The model under review builds one solid part; all positions refer to its coordinate system, in mm. A direction names the side the tool comes from. Give positions to 0.01 mm unless a question says otherwise; leave off trailing zeros. Order: outer loops, then holes, each group sorted by start corner. A loop starts at its lowest first (then second) coordinate and runs counter-clockwise, first axis right, second up.
Autodesk Inventor part; units mm, degrees
ref_plane "Work Plane1" through (-54.875, -108.1, -1.5875) normal (1, 0, 0) x (0, 1, 0)
ref_plane "YZ Plane" through (0, 0, 0) normal (1, 0, 0) x (0, 1, 0)
ref_plane "XZ Plane" through (0, 0, 0) normal (0, 1, 0) x (-1, 0, 0)
sketch "Sketch1" plane through (0, 0, 0) normal (0, 0, 1) x (1, 0, 0)
  line L0 (-1.5875, 0) -> (-1.5875, -108.1)
  line L1 (-54.875, 0) -> (-1.5875, 0)
  line L2 (-54.875, 0) -> (-54.875, -59)
  line L3 (-54.875, -59) -> (-18.9375, -59)
  arc A0 (-18.9375, -75) -> (-18.9375, -59) centre (-18.9375, -67) ccw
  line L4 (-18.9375, -75) -> (-54.875, -75)
  line L5 (-54.875, -75) -> (-54.875, -108.1)
  line L6 (-54.875, -108.1) -> (-1.5875, -108.1)
  circle A1 centre (-18.9375, -67) radius 2
  circle A2 centre (-18.9375, -67) radius 2
  circle A3 centre (-18.9375, -67) radius 7.5
  line L7 (-6.1875, -79.75) -> (-31.6875, -79.75) construction
  line L8 (-31.6875, -79.75) -> (-31.6875, -54.25) construction
  line L9 (-31.6875, -54.25) -> (-6.1875, -54.25) construction
  line L10 (-6.1875, -54.25) -> (-6.1875, -79.75) construction
  line L11 (-18.9375, -79.75) -> (-18.9375, -54.25) construction
  line L12 (-31.6875, -67) -> (-6.1875, -67) construction
  circle A4 centre (-6.1875, -79.75) radius 1.5
  circle A5 centre (-31.6875, -79.75) radius 1.5
  circle A6 centre (-31.6875, -54.25) radius 1.5
  circle A7 centre (-6.1875, -54.25) radius 1.5
  circle A8 centre (-6.1875, -79.75) radius 2.6 construction
  circle A9 centre (-31.6875, -79.75) radius 2.6 construction
  circle A10 centre (-31.6875, -54.25) radius 2.6 construction
  circle A11 centre (-6.1875, -54.25) radius 2.6 construction
  line L13 (-3.5875, -79.75) -> (-3.5875, -54.25) construction
  arc A12 (-8.0517, -82.7122) -> (-3.5875, -77.4069) centre (-6.1875, -79.75) ccw
  arc A13 (-34.6497, -77.8858) -> (-29.8233, -82.7122) centre (-31.6875, -79.75) ccw
  arc A14 (-29.8233, -51.2878) -> (-34.6497, -56.1142) centre (-31.6875, -54.25) ccw
  arc A15 (-3.5875, -56.5931) -> (-8.0517, -51.2878) centre (-6.1875, -54.25) ccw
  line L14 (-8.0517, -82.7122) -> (-17.8722, -76.532)
  line L15 (-34.6497, -56.1142) -> (-28.4695, -65.9347)
  line L16 (-34.6497, -77.8858) -> (-28.4695, -68.0653)
  line L17 (-3.2253, -56.1142) -> (-9.4055, -65.9347)
  line L18 (-3.2253, -77.8858) -> (-9.4055, -68.0653)
  line L19 (-29.8233, -51.2878) -> (-20.0028, -57.468)
  line L20 (-8.0517, -51.2878) -> (-17.8722, -57.468)
  line L21 (-20.3773, -59) -> (-20.6867, -59.1936)
  line L22 (-29.8233, -82.7122) -> (-20.0028, -76.532)
  arc A16 (-20.0028, -57.468) -> (-17.8722, -57.468) centre (-18.9375, -55.7753) ccw
  arc A17 (-28.4695, -68.0653) -> (-28.4695, -65.9347) centre (-30.1622, -67) ccw
  arc A18 (-17.8722, -76.532) -> (-20.0028, -76.532) centre (-18.9375, -78.2247) ccw
  arc A19 (-9.4055, -65.9347) -> (-9.4055, -68.0653) centre (-7.7128, -67) ccw
  circle A20 centre (-18.9375, -67) radius 2.5
  circle A21 centre (-31.6875, -54.25) radius 2.6
  circle A22 centre (-6.1875, -79.75) radius 2.6
  circle A23 centre (-6.1875, -54.25) radius 2.6
  circle A24 centre (-31.6875, -79.75) radius 2.6
  point P0 (0, 0)
  point P1 (-27.7991, -67)
  point P2 (-10.0759, -67)
  point P3 (-18.9375, -58.1384)
  point P4 (-18.9375, -75.8616)
  dimension "d2" = 5.2
  dimension "d1" = 3
  dimension "d4" = 2
  dimension "d5" = 2
  dimension "d6" = 2
  dimension "d9" = 0.5
extrude "Extrusion1" add sketch "Sketch1" along normal blind 4 contours L15 A14 L19 A16 L20 A15 L17 A19 L18 A12 L14 A18 L22 A13 L16 L4 A0 L3 | L3 A0 L4 L16 A17 L15 | A3 | A21 | A22 | A23 | A24
sketch "Sketch2" plane through (0, 0, 0) normal (0, 0, -1) x (-1, 0, 0)
  circle A0 centre (18.9375, -67) radius 7.5
  point P0 (0, 0)
extrude "Extrusion2" add sketch "Sketch2" along normal blind 1
sketch "Sketch3" plane through (0, 0, 0) normal (0, 0, -1) x (-1, 0, 0)
  line L0 (1.5875, 0) -> (1.5875, -108.1)
  line L1 (54.875, 0) -> (1.5875, 0)
  line L2 (54.875, 0) -> (54.875, -59)
  line L3 (54.875, -59) -> (18.9375, -59)
  arc A0 (18.9375, -59) -> (18.9375, -75) centre (18.9375, -67) ccw
  line L4 (18.9375, -75) -> (54.875, -75)
  line L5 (54.875, -75) -> (54.875, -108.1)
  line L6 (54.875, -108.1) -> (1.5875, -108.1)
  circle A1 centre (18.9375, -67) radius 7.5
  arc A2 (18.9375, -59) -> (18.9375, -75) centre (18.9375, -67) ccw
  circle A3 centre (18.9375, -67) radius 2.5
  arc A4 (22.7022, -74.0588) -> (22.7022, -59.9412) centre (18.9375, -67) ccw
  line L7 (53.2875, -108.1) -> (53.2875, 0)
  line L8 (54.875, 0) -> (54.875, -108.1)
  line L9 (53.2875, -59) -> (22.9375, -59)
  line L10 (18.9375, -59) -> (18.9375, -75)
  line L11 (22.9375, -75) -> (53.2875, -75)
  line L12 (53.2875, -75) -> (53.2875, -59)
  arc A5 (22.9375, -59) -> (22.7022, -59.9412) centre (22.9375, -59.5) ccw
  arc A6 (22.7022, -74.0588) -> (22.9375, -75) centre (22.9375, -74.5) ccw
  circle A7 centre (31.6875, -54.25) radius 2.6
  circle A8 centre (6.1875, -79.75) radius 2.6
  circle A9 centre (6.1875, -54.25) radius 2.6
  circle A10 centre (31.6875, -79.75) radius 2.6
  point P0 (0, 0)
  dimension "d12" = 0.5
extrude "Extrusion3" add sketch "Sketch3" along normal blind 2 contours L7 L4 A6 A4 A5 L3
sketch "Sketch4" plane through (-53.2875, -75, 0) normal (-1, 0, 0) x (0, 0, 1)
  line L0 (-1.5875, 75) -> (-1.5875, -33.1)
  line L1 (0, -33.1) -> (0, 75)
  line L2 (0, 15.0588) -> (0, 16)
  line L3 (0, 0) -> (-2, 0)
  line L4 (0, 16) -> (-1.5875, 16)
  line L5 (-1.5875, 16) -> (-1.5875, 0)
  line L6 (-1.5875, 0) -> (0, 0)
  line L7 (0, 0) -> (0, 16)
ref_plane "Work Plane1" through (-54.875, -108.1, -1.5875) normal (1, 0, 0) x (0, 1, 0)
extrude "Extrusion4" add sketch "Sketch4" along normal up to surface (1.5875 mm away)
sketch "Sketch5" plane through (0, 0, 4) normal (0, 0, 1) x (1, 0, 0)
  arc A0 (-28.4695, -68.0653) -> (-28.4695, -65.9347) centre (-30.1622, -67) ccw
  line L0 (-28.4695, -68.0653) -> (-34.6497, -77.8858)
  arc A1 (-34.6497, -77.8858) -> (-29.8233, -82.7122) centre (-31.6875, -79.75) ccw
  line L1 (-29.8233, -82.7122) -> (-20.0028, -76.532)
  arc A2 (-17.8722, -76.532) -> (-20.0028, -76.532) centre (-18.9375, -78.2247) ccw
  line L2 (-17.8722, -76.532) -> (-8.0517, -82.7122)
  arc A3 (-8.0517, -82.7122) -> (-3.2253, -77.8858) centre (-6.1875, -79.75) ccw
  line L3 (-3.2253, -77.8858) -> (-9.4055, -68.0653)
  arc A4 (-9.4055, -65.9347) -> (-9.4055, -68.0653) centre (-7.7128, -67) ccw
  line L4 (-9.4055, -65.9347) -> (-3.2253, -56.1142)
  arc A5 (-3.2253, -56.1142) -> (-8.0517, -51.2878) centre (-6.1875, -54.25) ccw
  line L5 (-8.0517, -51.2878) -> (-17.8722, -57.468)
  arc A6 (-20.0028, -57.468) -> (-17.8722, -57.468) centre (-18.9375, -55.7753) ccw
  line L6 (-20.0028, -57.468) -> (-29.8233, -51.2878)
  arc A7 (-29.8233, -51.2878) -> (-34.6497, -56.1142) centre (-31.6875, -54.25) ccw
  line L7 (-34.6497, -56.1142) -> (-28.4695, -65.9347)
  circle A8 centre (-18.9375, -67) radius 2.5
  circle A9 centre (-6.1875, -54.25) radius 1.5
  circle A10 centre (-31.6875, -54.25) radius 1.5
  circle A11 centre (-31.6875, -79.75) radius 1.5
  circle A12 centre (-6.1875, -79.75) radius 1.5
  circle A13 centre (-31.6875, -79.75) radius 3.5
  circle A14 centre (-31.6875, -54.25) radius 1.5
  circle A15 centre (-31.6875, -54.25) radius 3.5
  circle A16 centre (-6.1875, -79.75) radius 3.5
  arc A17 (-3.2253, -56.1142) -> (-8.0517, -51.2878) centre (-6.1875, -54.25) ccw
  circle A18 centre (-6.1388, -54.2188) radius 3.5
  point P0 (0, 0)
  point P1 (-34.6497, -56.1142)
  point P2 (-29.8233, -51.2878)
  point P3 (-2.2565, -55.1629)
  point P4 (-3.2253, -77.8858)
  point P5 (-8.0517, -82.7122)
  point P6 (-29.8233, -82.7122)
  point P7 (-3.4179, -56.4203)
extrude "Extrusion5" cut sketch "Sketch5" against normal blind 2 contours A13 A1 | A7 A15 | A16 A3 | A5 L4 A18 picked at (-4.1737, -56.2279)
fillet "Fillet1" radius 1 10 edges at (-8.0517, -82.7122, 3) (-3.2253, -77.8858, 3) (-3.2253, -56.1142, 1) (-8.0517, -51.2878, 1) (-29.8233, -51.2878, 3) (-34.6497, -56.1142, 3) (-34.6497, -77.8858, 3) (-29.8233, -82.7122, 3) (-3.4179, -56.4203, 3) (-8.0517, -51.2878, 3)
sketch "Sketch6" plane through (0, 0, 0) normal (0, 0, 1) x (1, 0, 0)
  line L0 (-32.8336, -59) -> (-28.4695, -65.9347)
  line L1 (-32.8336, -59) -> (-54.875, -59)
  line L2 (-54.875, -75) -> (-54.875, -59)
  line L3 (-32.8336, -75) -> (-54.875, -75)
  line L4 (-28.4695, -68.0653) -> (-32.8336, -75)
  arc A0 (-28.4695, -68.0653) -> (-28.4695, -65.9347) centre (-30.1622, -67) ccw
  line L5 (-53.2875, 0) -> (-53.2875, -108.1)
  line L6 (-35.6304, -72.5101) -> (-44.525, -72.5101)
  line L7 (-46.525, -70.5101) -> (-46.525, -63.4899)
  line L8 (-44.525, -61.4899) -> (-35.6304, -61.4899)
  line L9 (-33.6304, -63.4899) -> (-33.6304, -70.5101)
  line L10 (-28.1622, -67) -> (-54.875, -67) construction
  line L11 (-54.875, -59) -> (-54.875, -75) construction
  line L12 (-48.525, -39.75) -> (-48.525, -93.75) construction
  arc A1 (-35.6304, -72.5101) -> (-33.6304, -70.5101) centre (-35.6304, -70.5101) ccw
  arc A2 (-46.525, -70.5101) -> (-44.525, -72.5101) centre (-44.525, -70.5101) ccw
  arc A3 (-44.525, -61.4899) -> (-46.525, -63.4899) centre (-44.525, -63.4899) ccw
  arc A4 (-33.6304, -63.4899) -> (-35.6304, -61.4899) centre (-35.6304, -63.4899) ccw
  point P0 (0, 0)
  dimension "d20" = 2
  dimension "d21" = 2
extrude "Extrusion6" cut sketch "Sketch6" against normal through all contours L6 A2 L7 A3 L8 A4 L9 A1
properties part number "TurretBase"
Item 1: Take a section at B-B (z = 2.8). Give the boundary of the cut face in (x, y).
Values found:
outline: (-32.66, -74.72) arc R1 ccw to (-31.78, -76.25) arc R3.5 cw to (-28.19, -79.85) arc R1 ccw to (-26.66, -80.72) - (-20, -76.53) arc R2 cw to (-17.87, -76.53) - (-11.22, -80.72) arc R1 ccw to (-9.69, -79.85) arc R3.5 cw to (-6.09, -76.25) arc R1 ccw to (-5.22, -74.72) - (-9.41, -68.07) arc R2 cw to (-9.41, -65.93) - (-5.2, -59.25) arc R1 ccw to (-6.07, -57.72) arc R3.5 cw to (-9.64, -54.12) arc R1 ccw to (-11.17, -53.25) - (-17.87, -57.47) arc R2 cw to (-20, -57.47) - (-26.66, -53.28) arc R1 ccw to (-28.19, -54.15) arc R3.5 cw to (-31.78, -57.75) arc R1 ccw to (-32.66, -59.28) - (-28.47, -65.93) arc R2 cw to (-28.47, -68.07) - close; hole circle Ø5 at (-18.94, -67)
Item 2: Draft analysis for pull direction X (two halves, no side actions). For faces 6 (the cylindrical face through (-34.2, -62.09, -0.99)), 7 (the flat face through (-6.96, -71.95, 1.97)), 8 (the cylindrical face through (-32.88, -53.34, 0.99)), 9 (the flat face through (-39, -75, -1)), state which applies: released by +X, released by -X, zero draft, split by the parting line, or undercut.
Values found:
face 6: undercut
face 7: released by +X
face 8: undercut
face 9: zero draft
Item 3: Clearance check with flat-ended pins moving along their axes: pin 1 Ø1.8 at (x, y) = (-31.69, -79.75) entering from +Z; pin 2 Ø2 at (y, z) = (-70.5, 2) entering from -X; pin 3 Ø0.6 at (x, z) = (-39, -0.5) entering from +Y; pin 4 Ø4.5 at (x, y) = (-21, -64.5) entering from -Z. State where each tip first meets the part, or that it passes through.
Values found:
pin 1: passes through
pin 2: stops at x = -30.63
pin 3: stops at y = -59
pin 4: stops at z = -1
Item 4: For faces 1 (the flat face through (-33.63, -67, -1)), 2 (the flat face through (-6.96, -62.05, 1.97)), 3 (the flat face through (-23.89, -55.02, 1.97)), 4 (the cylindrical face through (-28.162, -66.984, 1.972)), 5 (the flat face through (-19, -67, 0)), list the 3-axis set-ups (+Z, -Z, +X, -X, +Y, -Y) from which the entire face can be reached by the end or side of a thin tool; tool diameter is ignored.
Values found:
face 1: +Z, -Z
face 2: +Z, -Z, +X
face 3: +Z, -Z, +Y
face 4: +Z, -X
face 5: +Z
Item 5: Take a section at A-A (y = -67). Give the boundary of the cut face in (x, z) (1 decimal), and give its area (3 significant figures).
Values found:
outline: (-54.9, -1.6) - (-53.3, -1.6) - (-53.3, -2) - (-46.5, -2) - (-46.5, 0) - (-54.9, 0) - close; (-33.6, -2) - (-26.9, -2) - (-26.9, 0) - (-26.4, 0) - (-26.4, -1) - (-11.4, -1) - (-11.4, 0) - (-9.7, 0) - (-9.7, 4) - (-16.4, 4) - (-16.4, 0) - (-21.4, 0) - (-21.4, 4) - (-28.2, 4) - (-28.2, 0) - (-33.6, 0) - close
area: 98.2 mm2
Item 6: Take a section at C-C (x = -13). Give the boundary of the cut face in (y, z), and give its area (3 significant figures).
Values found:
outline: (-79.6, 0) - (-71.58, 0) - (-71.58, -1) - (-62.42, -1) - (-62.42, 0) - (-54.4, 0) - (-54.4, 4) - (-79.6, 4) - close
area: 110 mm2
Item 7: Take a section at D-D (x = -49.5). Give the boundary of the cut face in (y, z).
Values found:
outline: (-75, -2) - (-59, -2) - (-59, 0) - (-75, 0) - close
Item 8: For line 1 (Y direction, x = -19, z = 0.7); line 2 (Z direction, x = -12, y = -54.5); line 3 (Z direction, x = -52, y = -73.5), list the stretches that pass through material, from the lowest coordinate up.
Values found:
line 1: y = -76.23 to -69.5, -64.5 to -57.77
line 2: z = 0 to 4
line 3: z = -2 to 0
